Part model, mm, in its own coordinate system. Face numbers are marked on the shaded views. Coordinates: 2 decimals unless noted, no trailing zeros. Order: outer loops, then holes, each group sorted by start corner. A loop starts at its lowest first (then second) coordinate and runs counter-clockwise, first axis right, second up.
1) Cut at A-A (x = -150). List the corners of the cut face in (y, z).
2) Mould opens along Z. For the marked faces 1, 2 and 3 say: +Z half, -Z half, draft (parallel to the pull), parting line (faces both ways), or undercut.
3) Wall check: L1, parallel to X at y = 2252.5, z = 6; L2, parallel to Y at x = -149, z = 13.25; L3, parallel to Y at x = -107.5, z = 5.75. Give the ranges that are in metal, low to high.
```python
from build123d import *

# Parameters (mm, degrees)
SKETCH1_W                = 149.100450595
SKETCH1_H                = 180.7
BOSS_EXTRUDE1_DEPTH      = 20
M6_CLEARANCE_HOLE1_D     = 6.6
M6_CLEARANCE_HOLE1_DEPTH = 36.6
M6_CLEARANCE_HOLE1_TIP   = 1.982840043


with BuildPart() as part:
    # Sketch1 → Boss-Extrude1 (new body)
    with BuildSketch(Plane.XY):
        with Locations((-126.988568818, 2276.898566852)):
            Rectangle(SKETCH1_W, SKETCH1_H)
    extrude(amount=BOSS_EXTRUDE1_DEPTH)

    # M6 Clearance Hole1
    with Locations(Plane.XY.offset(20)):
        with Locations((-149.488568817, 2307.048566852), (-104.488568817, 2307.048566852), (-104.488568817, 2250.048566852), (-149.488568817, 2250.048566852), (-137.988568818, 2362.548566852), (-137.988568818, 2324.548566852), (-115.988568818, 2324.548566852), (-115.988568818, 2362.548566852)):
            Hole(M6_CLEARANCE_HOLE1_D / 2, depth=M6_CLEARANCE_HOLE1_DEPTH)
            with Locations((0, 0, -(M6_CLEARANCE_HOLE1_DEPTH + M6_CLEARANCE_HOLE1_TIP / 2))):  # 118° drill point
                Cone(0, M6_CLEARANCE_HOLE1_D / 2, M6_CLEARANCE_HOLE1_TIP, mode=Mode.SUBTRACT)


solid = part.part
```
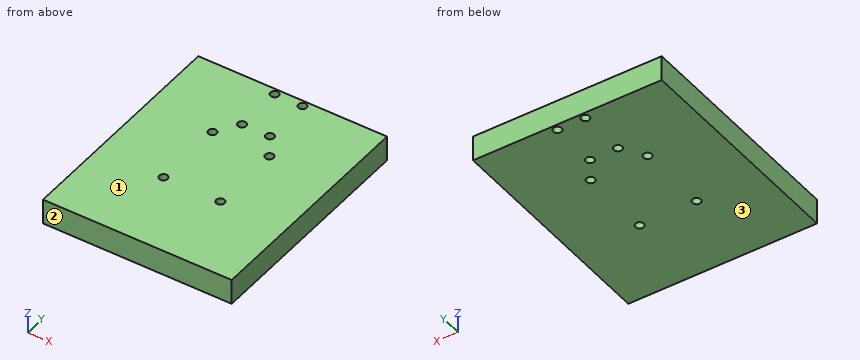
Geometry check:
1. outline: (2186.55, 0) - (2246.79, 0) - (2246.79, 20) - (2186.55, 20) - close; (2253.31, 0) - (2303.79, 0) - (2303.79, 20) - (2253.31, 20) - close; (2310.31, 0) - (2367.25, 0) - (2367.25, 20) - (2310.31, 20) - close
2. face 1: +Z half
2. face 2: draft
2. face 3: -Z half
3. L1: x = -201.54 to -151.7, -147.28 to -106.7, -102.28 to -52.44
3. L2: y = 2186.55 to 2246.78, 2253.31 to 2303.78, 2310.31 to 2367.25
3. L3: y = 2186.55 to 2248.7, 2251.4 to 2305.7, 2308.4 to 2367.25
